```python
from build123d import *

# Parameters (mm, degrees)
BOSS_EXTRUDE1_DEPTH      = 1.2
BOSS_EXTRUDE1_DEPTH_BACK = 4
SKETCH3_W                = 22.4
SKETCH3_H                = 1.5
BOSS_EXTRUDE2_DEPTH      = 1.2


with BuildPart() as part:
    # Sketch1 → Boss-Extrude1 (new, two sides: drawn at the far end of the back side and taken through both)
    with BuildSketch(Plane.XY.offset(-BOSS_EXTRUDE1_DEPTH_BACK)):
        with BuildLine():
            Line((-34.384444189, 19.919216619), (-7.984444189, 19.919216619))
            ThreePointArc((-7.984444189, 19.919216619), (8.465555811, 3.469216619), (-7.984444189, -12.980783381))
            Line((-7.984444189, -12.980783381), (-34.384444189, -12.980783381))
            ThreePointArc((-34.384444189, -12.980783381), (-50.834444189, 3.469216619), (-34.384444189, 19.919216619))
        make_face()
        with BuildLine():
            Line((-34.384444189, 18.719216619), (-7.984444189, 18.719216619))
            ThreePointArc((-7.984444189, 18.719216619), (7.265555811, 3.469216619), (-7.984444189, -11.780783381))
            Line((-7.984444189, -11.780783381), (-34.384444189, -11.780783381))
            ThreePointArc((-34.384444189, -11.780783381), (-49.634444189, 3.469216619), (-34.384444189, 18.719216619))
        make_face(mode=Mode.SUBTRACT)
    extrude(amount=BOSS_EXTRUDE1_DEPTH + BOSS_EXTRUDE1_DEPTH_BACK)

    # Sketch3 → Boss-Extrude2 (add)
    with BuildSketch(Plane.XY):
        with BuildLine():
            Line((-36.384444189, 17.07298448), (-36.384444189, 18.587500252))
            ThreePointArc((-36.384444189, 18.587500252), (-49.634444189, 3.469216619), (-36.384444189, -11.649067014))
            Line((-36.384444189, -11.649067014), (-36.384444189, -10.134551241))
            ThreePointArc((-36.384444189, -10.134551241), (-48.134444189, 3.469216619), (-36.384444189, 17.07298448))
        make_face()
        with BuildLine():
            Line((-36.384444189, 15.554848584), (-36.384444189, 17.07298448))
            ThreePointArc((-36.384444189, 17.07298448), (-48.134444189, 3.469216619), (-36.384444189, -10.134551241))
            Line((-36.384444189, -10.134551241), (-36.384444189, -8.616415346))
            ThreePointArc((-36.384444189, -8.616415346), (-46.634444189, 3.469216619), (-36.384444189, 15.554848584))
        make_face()
        with Locations((-21.184444189, 17.969216619)):
            Rectangle(SKETCH3_W, SKETCH3_H)
        with Locations((-21.184444189, 16.469216619)):
            Rectangle(SKETCH3_W, SKETCH3_H)
        with BuildLine():
            ThreePointArc((4.998717984, 11.469216619), (0.309606549, 16.266529711), (-5.984444189, 18.587500252))
            Line((-5.984444189, 18.587500252), (-5.984444189, 17.07298448))
            ThreePointArc((-5.984444189, 17.07298448), (-0.822090303, 15.206472977), (3.198690434, 11.469216619))
            Line((3.198690434, 11.469216619), (4.998717984, 11.469216619))
        make_face()
        with BuildLine():
            ThreePointArc((3.198690434, 11.469216619), (-0.822090303, 15.206472977), (-5.984444189, 17.07298448))
            Line((-5.984444189, 17.07298448), (-5.984444189, 15.554848584))
            ThreePointArc((-5.984444189, 15.554848584), (4.265555811, 3.469216619), (-5.984444189, -8.616415346))
            Line((-5.984444189, -8.616415346), (-5.984444189, -10.134551241))
            ThreePointArc((-5.984444189, -10.134551241), (-0.822090303, -8.268039739), (3.198690434, -4.530783381))
            Line((3.198690434, -4.530783381), (4.998717984, -4.530783381))
            ThreePointArc((4.998717984, -4.530783381), (7.265555811, 3.469216619), (4.998717984, 11.469216619))
            Line((4.998717984, 11.469216619), (3.198690434, 11.469216619))
        make_face()
        with BuildLine():
            ThreePointArc((-5.984444189, -11.649067014), (0.309606549, -9.328096472), (4.998717984, -4.530783381))
            Line((4.998717984, -4.530783381), (3.198690434, -4.530783381))
            ThreePointArc((3.198690434, -4.530783381), (-0.822090303, -8.268039739), (-5.984444189, -10.134551241))
            Line((-5.984444189, -10.134551241), (-5.984444189, -11.649067014))
        make_face()
        with Locations((-21.184444189, -9.530783381)):
            Rectangle(SKETCH3_W, SKETCH3_H)
        with Locations((-21.184444189, -11.030783381)):
            Rectangle(SKETCH3_W, SKETCH3_H)
    extrude(amount=BOSS_EXTRUDE2_DEPTH)


solid = part.part
```
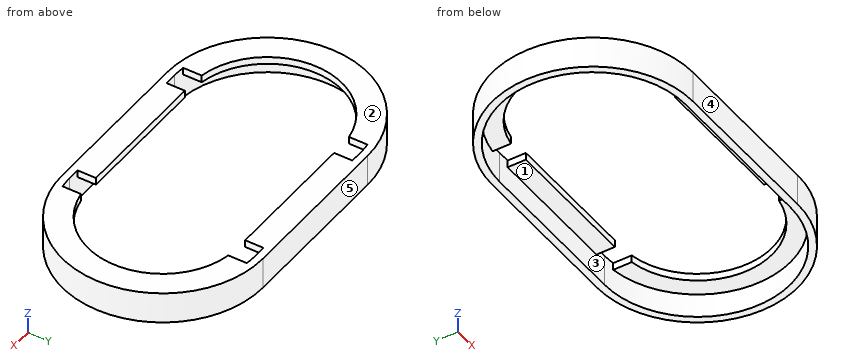
For this review, take the finished solid that the model builds, in its own axes (mm). Face numbers are marked on the shaded views. A direction names the side the tool comes from. Coordinates: 2 decimals unless noted, no trailing zeros. Loops run counter-clockwise (first coordinate to the right, second up) from the corner with the lowest first, then second, coordinate; pieces in that order, holes last.
1. Add section B-B, the plane z = -2.25. Give the boundary of the cut face in (x, y), then the cut area to 3 significant figures.
2. Add section D-D, the plane y = 10. Give the boundary of the cut face in (x, z).
3. Insertion check: P1, Ø0.6, axis at y = 17, z = 1, coming from the +X side; P2, Ø2, axis at x = -8, y = -6.5, coming from the +Z side; P3, Ø1, axis at y = -10.5, z = 1, coming from the -X side; P4, Ø0.6, axis at y = 16.5, z = 0.5, coming from the +X side. Each pin has a flat end and moves straight along its axis. Give the tip position at first contact, or say it passes through.
4. Add section C-C, the plane y = -11. Give the boundary of the cut face in (x, z), then the cut area to 3 significant figures.
5. For line 1 (Y direction, x = -8.5, z = -0.45); line 2 (X direction, y = 4, z = -2.15); line 3 (Y direction, x = -23.5, z = 0.3), list the stretches that pass through material, from the lowest coordinate up.
6. Mouldability with a two-part tool opening along Y and no side actions: class the marked faces 3, 4 and 5 as +Y half, -Y half, draft (parallel to the pull), parting line (faces both ways), or undercut.
7. Add section A-A, the plane x = -30. Give the boundary of the cut face in (y, z).
8. For the marked faces 1 and 2, list the 3-axis set-ups (+Z, -Z, +X, -X, +Y, -Y) from which the entire face can be reached by the end or side of a thin tool; tool diameter is ignored.
Result:
1. outline: (-34.38, -12.98) - (-7.98, -12.98) arc R16.45 ccw to (-7.98, 19.92) - (-34.38, 19.92) arc R16.45 ccw to start; hole (-34.38, -11.78) - (-7.98, -11.78) arc R15.25 ccw to (-7.98, 18.72) - (-34.38, 18.72) arc R15.25 ccw to start
1. area: 183 mm2
2. outline: (-49.48, -4) - (-48.17, -4) - (-48.17, 0) - (-44.75, 0) - (-44.75, 1.2) - (-49.48, 1.2) - close; (2.38, 0) - (5.8, 0) - (5.8, -4) - (7.11, -4) - (7.11, 1.2) - (2.38, 1.2) - close
3. P1: stops at x = 1.79
3. P2: passes through
3. P3: stops at x = -43.83
3. P4: stops at x = 2.43
4. outline: (-42.21, -4) - (-39.2, -4) - (-39.2, 0) - (-36.38, 0) - (-36.38, 1.2) - (-42.21, 1.2) - close; (-32.38, 0) - (-9.98, 0) - (-9.98, 1.2) - (-32.38, 1.2) - close; (-5.98, 0) - (-3.17, 0) - (-3.17, -4) - (-0.16, -4) - (-0.16, 1.2) - (-5.98, 1.2) - close
4. area: 64.9 mm2
5. line 1: y = -12.98 to -11.78, 18.72 to 19.92
5. line 2: x = -50.83 to -49.63, 7.26 to 8.46
5. line 3: y = -12.98 to -8.78, 15.72 to 19.92
6. face 3: undercut
6. face 4: -Y half
6. face 5: +Y half
7. outline: (-12.98, -4) - (-11.78, -4) - (-11.78, 0) - (-8.78, 0) - (-8.78, 1.2) - (-12.98, 1.2) - close; (15.72, 0) - (18.72, 0) - (18.72, -4) - (19.92, -4) - (19.92, 1.2) - (15.72, 1.2) - close
8. face 1: -Z
8. face 2: +Z, +X, -X, +Y, -Y
